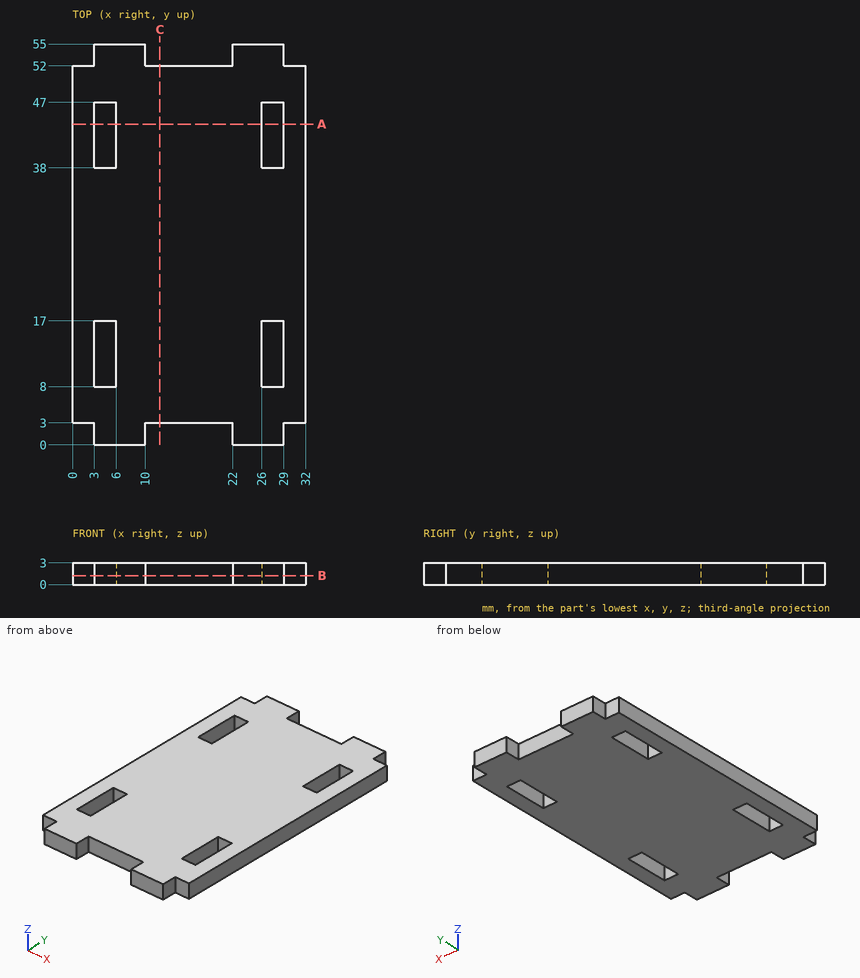
Geometry check sheet. Reference: drawing and pictorial views, mm from the part's lowest x, y, z. Give positions to 0.01 mm unless a question says otherwise; leave off trailing zeros. Write each loop counter-clockwise with the first axis right and the second up, starting at its lowest first coordinate (ties: lowest second). Pieces come first, ordered by that corner, then holes. Notation, with made-up numbers: (62, 9) -> (76, 9) arc R29 ccw to (76, 46) -> close; hole circle Ø7 at (86, -37.5). An arc over 180 degrees is marked (long way). One line per item, written item: value. Start each with the question number.
Item 1: Material ranges on probe 1 along Y at (x, z) = (26.5, 1.6); probe 2 along X at (y, z) = (41, 0.8); probe 3 along Y at (x, z) = (17, 0.3), recorded low to high. Write a range as from..to.
Item 2: Section check C-C on x = 12. Record the cut outline in (y, z), then the cut area to 3 significant figures.
Item 3: Section check A-A on y = 44. Record the cut outline in (x, z).
Item 4: Gauge pin test, flat ends, axial feed: pin 1 (0.9 mm diameter, centred on y = 54, z = 1, fed in from +X); pin 2 (2 mm diameter, centred on x = 20, y = 43, fed in from -Z). Record the tip position at first contact, or that the pin passes through.
Item 5: Section check B-B on z = 1.25. State how many separate pieces and enclosed holes the cut face has, then the cut area to 3 significant figures.
Results list:
1. probe 1: 0..8, 17..38, 47..55
1. probe 2: 0..3, 6..26, 29..32
1. probe 3: 3..52
2. outline: (3, 0) -> (52, 0) -> (52, 3) -> (3, 3) -> close
2. area: 147 mm²
3. outline: (0, 0) -> (3, 0) -> (3, 3) -> (0, 3) -> close; (6, 0) -> (26, 0) -> (26, 3) -> (6, 3) -> close; (29, 0) -> (32, 0) -> (32, 3) -> (29, 3) -> close
4. pin 1: x = 29
4. pin 2: z = 0
5. separate pieces: 1
5. enclosed holes: 4
5. area: 1,540 mm²
